Part model, mm, in its own coordinate system. A direction names the side the tool comes from. Coordinates: 2 decimals unless noted, no trailing zeros. Loops run counter-clockwise (first coordinate to the right, second up) from the corner with the lowest first, then second, coordinate; pieces in that order, holes last. Notation, with made-up numbers: (61.5, 42.5) - (65.5, 42.5) arc R14 cw to (65.5, 54.5) - close; hole circle Ø6 at (38.5, 88). An arc over 180 degrees is marked (long way). Answer as CSV lines item,"result".
from build123d import *

# Parameters (mm, degrees)
F1_DEPTH = 3
F2_W     = 10
F2_H     = 62
F3_DEPTH = 25


with BuildPart() as f1:
    # F0 (on Front) → F1 (new body)
    with BuildSketch(Plane.XZ):
        Polygon((17.5, -45), (17.5, 45), (-17.5, 45), (-17.5, -45), (-10, -55), (10, -55), align=None)
        with BuildLine():
            Line((4, -8), (4, -31))
            ThreePointArc((4, -31), (2.828427, -33.828427), (0, -35))
            ThreePointArc((0, -35), (-2.828427, -33.828427), (-4, -31))
            Line((-4, -31), (-4, -8))
            ThreePointArc((-4, -8), (-2.828427, -5.171573), (0, -4))
            ThreePointArc((0, -4), (2.828427, -5.171573), (4, -8))
        make_face(mode=Mode.SUBTRACT)
        with BuildLine():
            Line((4, 30), (4, 7))
            ThreePointArc((4, 7), (2.828427, 4.171573), (0, 3))
            ThreePointArc((0, 3), (-2.828427, 4.171573), (-4, 7))
            Line((-4, 7), (-4, 30))
            ThreePointArc((-4, 30), (-2.828427, 32.828427), (0, 34))
            ThreePointArc((0, 34), (2.828427, 32.828427), (4, 30))
        make_face(mode=Mode.SUBTRACT)
    extrude(amount=F1_DEPTH)

    # F2 (on face) → F3 (cut)
    with BuildSketch(Plane.XZ.offset(3)):
        with Locations((-12.5, 14)):
            Rectangle(F2_W, F2_H)
        with Locations((12.5, 14)):
            Rectangle(F2_W, F2_H)
    extrude(amount=-F3_DEPTH, mode=Mode.SUBTRACT)


solid = f1.part
Q1. Saw through at C-C (x = 2). Give the cut face in (y, z), then the cut area to 3 significant figures.
Results:
outline,"(-3, -55) - (0, -55) - (0, -34.46) - (-3, -34.46) - close; (-3, -4.54) - (0, -4.54) - (0, 3.54) - (-3, 3.54) - close; (-3, 33.46) - (0, 33.46) - (0, 45) - (-3, 45) - close"
area,"120 mm^2"
Q2. Which spindle directions (+Z, -Z, +X, -X, +Y, -Y) get a long thin tool onto all of the face, cutting with end or side? Do faces 1 (the face through (17.5, -1, -31)), 2 (the face through (4, -1, -19)), 3 (the face through (12, -2, -17)). Say none if no direction does.
Results:
face 1,"+Z, -Z, +X, +Y, -Y"
face 2,"+Y, -Y"
face 3,"+Z, +X, +Y, -Y"
Q3. Saw through at A-A (z = -15). Give the cut face in (x, y).
Results:
outline,"(-7.5, -3) - (-4, -3) - (-4, 0) - (-7.5, 0) - close; (4, -3) - (7.5, -3) - (7.5, 0) - (4, 0) - close"
Q4. Saw through at D-D (z = 5.5). Give the cut face in (x, y).
Results:
outline,"(-7.5, -3) - (-3.71, -3) - (-3.71, 0) - (-7.5, 0) - close; (3.71, -3) - (7.5, -3) - (7.5, 0) - (3.71, 0) - close"
Q5. Wall check: L1, parallel to X at y = -0.4, z = 10.5; L2, parallel to Z at x = -2, y = -0.35; L3, parallel to Z at x = 3, y = -0.45. Give the ranges that are in metal, low to high.
Results:
L1,"x = -7.5 to -4, 4 to 7.5"
L2,"z = -55 to -34.46, -4.54 to 3.54, 33.46 to 45"
L3,"z = -55 to -33.65, -5.35 to 4.35, 32.65 to 45"
Q6. Saw through at B-B (y = -0.5). Give the cut face in (x, z), then the cut area to 3 significant figures.
Results:
outline,"(-17.5, -45) - (-10, -55) - (10, -55) - (17.5, -45) - (17.5, -17) - (7.5, -17) - (7.5, 45) - (-7.5, 45) - (-7.5, -17) - (-17.5, -17) - close; hole (-4, -31) arc R4 ccw to (4, -31) - (4, -8) arc R4 ccw to (-4, -8) - close; hole (-4, 7) arc R4 ccw to (4, 7) - (4, 30) arc R4 ccw to (-4, 30) - close"
area,"1,720 mm^2"
Q7. Two-plate mould, pull along X, no slides. Class faces 4 (the face through (-4, -1, 18)), 5 (the face through (-7.5, -2, 14)), 6 (the face through (4, -1, 19)), 7 (the face through (-13, -2, -17)): released by +X, released by -X, zero draft, split by the parting line, or undercut.
Results:
face 4,"undercut"
face 5,"released by -X"
face 6,"undercut"
face 7,"zero draft"
Q8. Flat gauge pins, fed straight in: pin 1 (1.5 mm diameter, centred on y = -2, z = 15, fed in from -X); pin 2 (0.9 mm diameter, centred on x = 13.5, y = -1.5, fed in from +Z); pin 3 (1.5 mm diameter, centred on y = -2, z = 13.5, fed in from +X). Where does each tip first touch, or does it go through?
Results:
pin 1,"stops at x = -7.5"
pin 2,"stops at z = -17"
pin 3,"stops at x = 7.5"
